```python
from build123d import *

# Parameters (mm, degrees)
SKETCH1_R               = 19
SKETCH1_R_2             = 17
CUT_EXTRUDE1_DEPTH      = 93.881645167
CUT_EXTRUDE1_DEPTH_BACK = 93.881645167
SKETCH3_R               = 17


with BuildPart() as part:
    # Sweep1: sweep along a path in Sketch2
    with BuildLine(Plane(origin=(0, 0, 0), x_dir=(1, 0, 0), z_dir=(0, 1, 0))) as sweep1_path:
        Line((0, 0), (0, 60))
        Line((0, 60), (-45, 60))
    # Sketch1 → Sweep1 (sweep)
    with BuildSketch(Plane.XY):
        Circle(SKETCH1_R)
        Circle(SKETCH1_R_2, mode=Mode.SUBTRACT)
    sweep(path=sweep1_path.line, transition=Transition.RIGHT)

    # Mirror1: part across plane


with BuildPart() as part_1:
    add(part.part)
    add(part.part.mirror(Plane(origin=(0, 0, 0), x_dir=(0, 0, 1), z_dir=(1, 0, 0))))

    # Sketch3 → Cut-Extrude1 (cut, two sides: drawn at the far end of the back side and taken through both)
    with BuildSketch(Plane(origin=(0, 0, 0), x_dir=(0, 0, -1), z_dir=(1, 0, 0)).offset(-CUT_EXTRUDE1_DEPTH_BACK)):
        with Locations((60, 0)):
            Circle(SKETCH3_R)
    extrude(amount=CUT_EXTRUDE1_DEPTH + CUT_EXTRUDE1_DEPTH_BACK, mode=Mode.SUBTRACT)


solid = part_1.part
```
Geometry check sheet. Reference: the model listing, model coordinates, mm. A direction names the side the tool comes from. Give positions to 0.01 mm unless a question says otherwise; leave off trailing zeros. Order: outer loops, then holes, each group sorted by start corner. A loop starts at its lowest first (then second) coordinate and runs counter-clockwise, first axis right, second up. Notation, with made-up numbers: (64.5, 46) - (86.5, 46) arc R28 cw to (86.5, 70) - close; hole circle Ø6 at (30, 22). An arc over 180 degrees is marked (long way). Answer in a Markdown table with one row per item. Add a question column.
Q1. Gauge pin test, flat ends, axial feed: pin 1 (8 mm diameter, centred on x = -16.5, z = -25, fed in from -Y); pin 2 (12 mm diameter, centred on x = 26.5, z = -42, fed in from -Y); pin 3 (2 mm diameter, centred on x = 26, z = -53, fed in from -Y). Record the tip position at first contact, or that the pin passes through.
Q2. Cross-section at B-B, the plane z = -63. Enter the section's corners in (x, y).
Q3. Tool access check on faces 1 (the flat face through (45, 10, -74)), 2 (the cylindrical face through (-18.98, -0.84, -23.75)). Record the directions out of +Z, -Z, +X, -X, +Y, -Y that give a thin tool (end or side, any length) a straight path to the whole face; none if there is none.
Q4. Material ranges on probe 1 along X at (y, z) = (0, -22); probe 2 along Z at (x, y) = (28, -9), recorded low to high. Write a range as from..to.
Q5. Cross-section at C-C, the plane x = 0. Enter the section's corners in (y, z).
Q6. Mould release check, pull along Y, two halves, no side actions. Record for faces 3 (the cylindrical face through (0.63, 7.28, -77.55)), 4 (the cylindrical face through (-0.63, -6.511, -75.704)), 5 (the flat face through (-14, -10, 0)): pulls with the +Y half, pulls with the -Y half, needs draft (parallel to the pull), parting line crosses it, or undercut.
Q7. Cross-section at D-D, the plane z = -29.5. Enter the section's corners in (x, y).
Q8. Cross-section at A-A, the plane y = 0. Enter the section's corners in (x, z), then the cut area to 3 significant figures.
Check values:
| question | item | result |
|---|---|---|
| 1 | pin 1 | stops at y = -14.31 |
| 1 | pin 2 | stops at y = -14.73 |
| 1 | pin 3 | stops at y = -18.03 |
| 2 | outline | (-45, -18.76) - (45, -18.76) - (45, -16.73) - (-45, -16.73) - close; (-45, 16.73) - (45, 16.73) - (45, 18.76) - (-45, 18.76) - close |
| 3 | face 1 | +Z, -Z, +X, +Y, -Y |
| 3 | face 2 | +Z |
| 4 | probe 1 | x = -19..-17, 17..19 |
| 4 | probe 2 | z = -76.73..-74.42, -45.58..-43.27 |
| 5 | outline | (-19, -60) arc R19 ccw to (19, -60) - (19, 0) - (17, 0) - (17, -60) arc R17 cw to (-17, -60) - (-17, 0) - (-19, 0) - close |
| 6 | face 3 | parting line crosses it |
| 6 | face 4 | undercut |
| 6 | face 5 | needs draft |
| 7 | outline | circle Ø38 at (0, 0); hole circle Ø34 at (0, 0) |
| 8 | outline | (-45, -79) - (45, -79) - (45, -77) - (-45, -77) - close; (-45, -43) - (-17, -43) - (-17, 0) - (-19, 0) - (-19, -41) - (-45, -41) - close; (17, -43) - (45, -43) - (45, -41) - (19, -41) - (19, 0) - (17, 0) - close |
| 8 | area | 456 mm^2 |
